```python
from build123d import *

# Parameters (mm, degrees)
SKETCH1_R           = 6.5
SKETCH1_R_2         = 5.58
BOSS_EXTRUDE1_DEPTH = 5
BOSS_EXTRUDE2_START = 1
SKETCH2_R           = 7
SKETCH2_R_2         = 6.5
BOSS_EXTRUDE2_DEPTH = 1
CHAMFER1_SIZE       = 0.7


with BuildPart() as part:
    # Sketch1 → Boss-Extrude1 (new, symmetric)
    with BuildSketch(Plane.XY):
        Circle(SKETCH1_R)
        Circle(SKETCH1_R_2, mode=Mode.SUBTRACT)
    extrude(amount=BOSS_EXTRUDE1_DEPTH, both=True)

    # Sketch2 → Boss-Extrude2 (add)
    with BuildSketch(Plane.XY.offset(-5).offset(BOSS_EXTRUDE2_START)):
        Circle(SKETCH2_R)
        Circle(SKETCH2_R_2, mode=Mode.SUBTRACT)
    boss_extrude2 = extrude(amount=-BOSS_EXTRUDE2_DEPTH)

    # Mirror1: Boss-Extrude2 across plane
    add(boss_extrude2.mirror(Plane.XY))

    # Chamfer1
    # the kernel refuses this chamfer: 0.7 mm, written as the material it takes off along each edge
    with BuildSketch(Plane(origin=(0, 0, 4), x_dir=(1, 0, 0), z_dir=(0, -1, 0))) as chamfer1_piece_1_section:
        Polygon((7 - CHAMFER1_SIZE, 0), (7, CHAMFER1_SIZE), (7, 0), align=None)
    chamfer1_piece_1 = revolve(axis=Axis((0, 0, 4), (0, 0, 1)), mode=Mode.PRIVATE)
    chamfer1_piece_1 = chamfer1_piece_1 - Plane(origin=(0, 0, 4.444446297), x_dir=(1, 0, 0), z_dir=(0, 0, 1)) * Cylinder(6.5, 29, mode=Mode.PRIVATE)
    add(chamfer1_piece_1, mode=Mode.SUBTRACT)
    with BuildSketch(Plane(origin=(0, 0, -4), x_dir=(1, 0, 0), z_dir=(0, -1, 0))) as chamfer1_piece_2_section:
        Polygon((7 - CHAMFER1_SIZE, 0), (7, -CHAMFER1_SIZE), (7, 0), align=None)
    chamfer1_piece_2 = revolve(axis=Axis((0, 0, -4), (0, 0, 1)), mode=Mode.PRIVATE)
    chamfer1_piece_2 = chamfer1_piece_2 - Plane(origin=(0, 0, -4.444446297), x_dir=(1, 0, 0), z_dir=(0, 0, 1)) * Cylinder(6.5, 29, mode=Mode.PRIVATE)
    add(chamfer1_piece_2, mode=Mode.SUBTRACT)


solid = part.part
```
The listing builds one solid part. Answer for the finished solid, in the listing's coordinates (mm). Coordinates: 2 decimals unless noted, no trailing zeros. Order: outer loops, then holes, each group sorted by start corner. A loop starts at its lowest first (then second) coordinate and runs counter-clockwise, first axis right, second up. Notation, with made-up numbers: M -31.5,35.25 L -22.5,35.25 A26 ccw -22.5,69.25 Z; hole C 62.5,62.5 d8. An arc over 180 degrees is marked long. Answer as a JSON object with one key per item and string values. Group by question number.
1. Determine the mould class of faces 1 (the flat face through (-5, -3, -5)), 2 (the cylindrical face through (3.23, -6.21, 4.85)), 3 (the cylindrical face through (-5.158, -3.955, 0.059)) for opening direction Z: released by +Z, released by -Z, zero draft, split by the parting line, or undercut.
2. Section A-A on x = 0 is taken. Write down the section's boundary in (y, z).
3. Flat-ended cylindrical pins translate along their axes: P1, Ø3, axis at x = 4, y = 3.5, coming from the +Z side; P2, Ø3, axis at x = 1, z = -2.5, coming from the -Y side; P3, Ø1.5, axis at y = -3.5, z = 2.5, coming from the +X side; P4, Ø3, axis at x = -2, z = 0, coming from the +Y side. Find the tip coordinate at first contact, or state that the pin passes through.
4. Section C-C on z = 1.25 is taken. Write down the section's boundary in (x, y).
5. Straight lines are drawn through the part: line 1 (Y direction, x = 0, z = 2.5); line 2 (Y direction, x = -3, z = 1.75); line 3 (X direction, y = 0.5, z = -3). For each, find the intervals that lie inside material, in ascending order.
Values follow:
{
 "1": {"face 1": "released by -Z", "face 2": "zero draft", "face 3": "undercut"},
 "2": {"outline": "M -7,-5 L -5.58,-5 L -5.58,5 L -7,5 L -7,4.7 L -6.5,4.2 L -6.5,-4.2 L -7,-4.7 Z; M 5.58,-5 L 7,-5 L 7,-4.7 L 6.5,-4.2 L 6.5,4.2 L 7,4.7 L 7,5 L 5.58,5 Z"},
 "3": {"P1": "z = 5", "P2": "y = -6.5", "P3": "x = 5.89", "P4": "y = 6.48"},
 "4": {"outline": "C 0,0 d13; hole C 0,0 d11.16"},
 "5": {"line 1": "-6.5 to -5.58, 5.58 to 6.5", "line 2": "-5.77 to -4.7, 4.7 to 5.77", "line 3": "-6.48 to -5.56, 5.56 to 6.48"}
}
